```python
from build123d import *

# Parameters (mm, degrees)
F1_DEPTH = 25.4


with BuildPart() as f1:
    # F0 (on Front) → F1 (new body)
    with BuildSketch(Plane.XZ):
        with BuildLine():
            Line((-50.8, 0), (0, 0))
            Line((0, 0), (0, 1.778))
            Line((0, 1.778), (-4.826, 1.778))
            ThreePointArc((-4.826, 1.778), (-6.4135, 2.203369), (-7.575631, 3.3655))
            Line((-7.575631, 3.3655), (-34.961952, 50.8))
            Line((-34.961952, 50.8), (-50.8, 50.8))
            Line((-50.8, 50.8), (-50.8, 0))
        make_face()
    extrude(amount=F1_DEPTH)

    # F2: F1 across plane


with BuildPart() as f1_1:
    add(f1.part)
    add(f1.part.mirror(Plane.YZ))


solid = f1_1.part
```
For this review, take the finished solid that the model builds, in its own axes (mm). A direction names the side the tool comes from. Round coordinates to 2 decimals unless told otherwise and drop trailing zeros. Write each loop counter-clockwise with the first axis right and the second up, starting at its lowest first coordinate (ties: lowest second). Pieces come first, ordered by that corner, then holes. Notation, with made-up numbers: (32, 42.5) - (50, 42.5) arc R27 cw to (50, 76.5) - close; hole circle Ø11 at (63.5, 81.5). An arc over 180 degrees is marked (long way). Answer as CSV lines item,"result". Start each with the question number.
(1) For line 1 (X direction, y = -23, z = 30.5); line 2 (X direction, y = -3.5, z = 33); line 3 (Z direction, x = 2, y = -14), list the stretches that pass through material, from the lowest coordinate up.
(2) Add section A-A, the plane z = 9.5. State the section outline as (x, y) points.
(3) Machinability: for faces 1 (the flat face through (-43, -13, 50.8)), 2 (the cylindrical face through (6.39, -12.52, 2.19)), which of the approach directions +Z, -Z, +X, -X, +Y, -Y give a long, thin tool a straight path to every point of the face, cutting with its end or side? Answer none if there is none.
(4) For pin 1 (3 mm diameter, centred on x = -31, y = -5.5, fed in from -Z); pin 2 (10.5 mm diameter, centred on x = 0.5, y = -11.5, fed in from +Z); pin 3 (1.5 mm diameter, centred on x = 1.5, y = -6, fed in from +Z); pin 4 (10 mm diameter, centred on x = 16, y = -13.5, fed in from +Z), all flat-tipped, find the tip position at first contact; note any pin that passes through.
(5) Add section D-D, the plane x = -3.5. State the section outline as (y, z) points, plus the area to 3 significant figures.
(6) Add section C-C, the plane z = 35.5. State the section outline as (x, y) points, plus the area to 3 significant figures.
(7) Mouldability with a two-part tool opening along X and no side actions: class faces 3 (the flat face through (50.8, -13, 26)), 4 (the flat face through (12, 0, 9)), 5 (the cylindrical face through (-6.39, -12.52, 2.19)), 6 (the flat face through (-50.8, -13, 26)) as +X half, -X half, draft (parallel to the pull), parting line (faces both ways), or undercut.
From the geometry:
1,line 1,"x = -50.8 to -23.24, 23.24 to 50.8"
1,line 2,"x = -50.8 to -24.69, 24.69 to 50.8"
1,line 3,"z = 0 to 1.78"
2,outline,"(-50.8, -25.4) - (-11.12, -25.4) - (-11.12, 0) - (-50.8, 0) - close; (11.12, -25.4) - (50.8, -25.4) - (50.8, 0) - (11.12, 0) - close"
3,face 1,"+Z, +X, -X, +Y, -Y"
3,face 2,"+Z, +Y, -Y"
4,pin 1,"stops at z = 0"
4,pin 2,"stops at z = 1.92"
4,pin 3,"stops at z = 1.78"
4,pin 4,"stops at z = 26.62"
5,outline,"(-25.4, 0) - (0, 0) - (0, 1.78) - (-25.4, 1.78) - close"
5,area,"45.2 mm²"
6,outline,"(-50.8, -25.4) - (-26.13, -25.4) - (-26.13, 0) - (-50.8, 0) - close; (26.13, -25.4) - (50.8, -25.4) - (50.8, 0) - (26.13, 0) - close"
6,area,"1,250 mm²"
7,face 3,"+X half"
7,face 4,"draft"
7,face 5,"undercut"
7,face 6,"-X half"
